Autodesk Inventor part; units mm, degrees
ref_plane "YZ Plane" through (0, 0, 0) normal (1, 0, 0) x (0, 1, 0)
ref_plane "XZ Plane" through (0, 0, 0) normal (0, 1, 0) x (-1, 0, 0)
ref_plane "XY Plane" through (0, 0, 0) normal (0, 0, 1) x (1, 0, 0)
sketch "Sketch1" plane through (0, 0, 0) normal (0, 1, 0) x (-1, 0, 0)
  circle A0 centre (0, 0) radius 2
  dimension "d0" = 4
extrude "Extrusion1" add sketch "Sketch1" along normal blind 15
sketch "Sketch2" plane through (0, 15, 0) normal (0, 1, 0) x (1, 0, 0)
  circle A0 centre (0, 0) radius 2
  circle A1 centre (0, 0) radius 3.5
  dimension "d3" = 7
extrude "Extrusion2" add sketch "Sketch2" along normal blind 4 contours A0 | A1
sketch "Sketch3" plane through (0, 19, 0) normal (0, 1, 0) x (1, 0, 0)
  circle A0 centre (0, 0) radius 3.5
  line L0 (0, 1.8475) -> (1.6, 0.9238)
  line L1 (1.6, 0.9238) -> (1.6, -0.9238)
  line L2 (1.6, -0.9238) -> (0, -1.8475)
  line L3 (0, -1.8475) -> (-1.6, -0.9238)
  line L4 (-1.6, -0.9238) -> (-1.6, 0.9238)
  line L5 (-1.6, 0.9238) -> (0, 1.8475)
  dimension "d6" = 1.6
extrude "Extrusion3" cut sketch "Sketch3" against normal blind 3 contours L0 L1 L2 L3 L4 L5
thread "Thread1"
chamfer "Chamfer1" distance 0.25 angle 45 1 edges at (2, 0, 0)
properties part number "SHCS4x15"
CAD build for the part. Positions are in the model's coordinates, mm. A direction names the side the tool comes from. Coordinates: 2 decimals unless noted, no trailing zeros. Loops run counter-clockwise (first coordinate to the right, second up) from the corner with the lowest first, then second, coordinate; pieces in that order, holes last. Notation, with made-up numbers: (65.5, -26.75) - (102.5, -26.75) arc R23 ccw to (102.5, -17.75) - close; hole circle Ø9 at (-34, 44.25). An arc over 180 degrees is marked (long way). Return JSON: item names as keys, results as strings.
1. Band-saw the part on D-D (y = 3.5). Give the cut face in (x, z), and give its area (3 significant figures).
Result:
{"outline": "circle Ø4 at (0, 0)", "area": "12.6 mm2"}
2. Mould opens along X. For faces 4 (the flat face through (2, 15, 2)), 5 (the cylindrical face through (3.233, 16.972, -1.341)), 6 (the flat face through (-1.6, 18, 0)) say: released by +X, released by -X, zero draft, split by the parting line, or undercut.
Result:
{"face 4": "zero draft", "face 5": "split by the parting line", "face 6": "undercut"}
3. 3-axis set-ups, long thin cutter, end or side, ignore diameter. For faces 1 (the cylindrical face through (0, 8, 2)), 2 (the flat face through (0, 0, 0)), 3 (the flat face through (-0.79, 17.52, 1.39)): which of +Z, -Z, +X, -X, +Y, -Y reach the whole face in a straight line?
Result:
{"face 1": "-Y", "face 2": "+Z, -Z, +X, -X, -Y", "face 3": "+Y"}
4. Probe L1, parallel to Y at x = 2.5, z = -0.5; L2, parallel to Y at x = -0.75, z = -1; L3, parallel to Z at x = -0.5, y = 11.25. List the from-to ranges inside material, lowest first. Write a range as from..to.
Result:
{"L1": "y = 15..19", "L2": "y = 0..16", "L3": "z = -1.94..1.94"}
5. Band-saw the part on C-C (x = -2.25). Give the cut face in (y, z), and give its area (3 significant figures).
Result:
{"outline": "(15, -2.68) - (19, -2.68) - (19, 2.68) - (15, 2.68) - close", "area": "21.4 mm2"}
6. Drop flat-ended pins along their axis: pin 1 (1 mm diameter, centred on x = 0.5, z = -0.5, fed in from +Y); pin 2 (1 mm diameter, centred on x = 0, y = 13, fed in from +Z). Give the stop position or say it passes through.
Result:
{"pin 1": "stops at y = 16", "pin 2": "stops at z = 2"}
7. Band-saw the part on B-B (y = 15.5). Give the cut face in (x, z), and give its area (3 significant figures).
Result:
{"outline": "circle Ø7 at (0, 0)", "area": "38.5 mm2"}
8. Band-saw the part on A-A (z = 0). Give the cut face in (x, y).
Result:
{"outline": "(-3.5, 15) - (-2, 15) - (-2, 0.25) - (-1.75, 0) - (1.75, 0) - (2, 0.25) - (2, 15) - (3.5, 15) - (3.5, 19) - (1.6, 19) - (1.6, 16) - (-1.6, 16) - (-1.6, 19) - (-3.5, 19) - close"}
